```python
from build123d import *

# Parameters (mm, degrees)
SKETCH1_W           = 6.35
SKETCH1_H           = 12.7
BOSS_EXTRUDE1_DEPTH = 2.54
SKETCH2_W           = 6.35
SKETCH2_H           = 0.127
BOSS_EXTRUDE2_DEPTH = 0.254
CUT_EXTRUDE1_DEPTH  = 10.404862359


with BuildPart() as part:
    # Sketch1 → Boss-Extrude1 (new body)
    with BuildSketch(Plane.XY):
        Rectangle(SKETCH1_W, SKETCH1_H)
    extrude(amount=BOSS_EXTRUDE1_DEPTH)

    # Sketch2 → Boss-Extrude2 (add)
    with BuildSketch(Plane.XY.offset(2.54)):
        with Locations((0, -6.2865)):
            Rectangle(SKETCH2_W, SKETCH2_H)
    boss_extrude2 = extrude(amount=BOSS_EXTRUDE2_DEPTH)

    # Mirror1: Boss-Extrude2 across plane
    add(boss_extrude2.mirror(Plane.ZX))

    # Sketch3 → Cut-Extrude1 (cut, through all)
    with BuildSketch(Plane(origin=(3.175, 0, 0), x_dir=(0, 0, -1), z_dir=(1, 0, 0))):
        Polygon((0, -6.35), (-2.286, -6.35), (0, 0), align=None)
    extrude(amount=-CUT_EXTRUDE1_DEPTH, mode=Mode.SUBTRACT)


solid = part.part
```
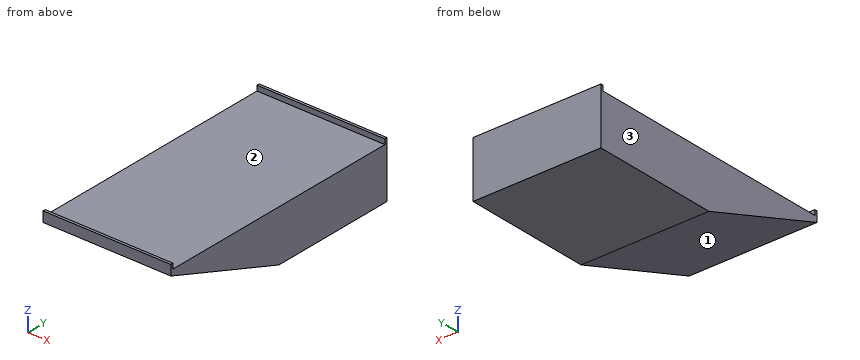
Work out the finished part from the listing and answer in its coordinate system (mm). Face numbers are marked on the shaded views. Round coordinates to 2 decimals unless told otherwise and drop trailing zeros. Loops run counter-clockwise (first coordinate to the right, second up) from the corner with the lowest first, then second, coordinate; pieces in that order, holes last. Notation, with made-up numbers: M 70,-40 L 119,-40 A32 ccw 119,-3 Z; hole C -10.75,0 d2. An arc over 180 degrees is marked long. One line per question, with ' | ' between items.
Q1. Consider line 1 along Z through (x, y) = (1.25, 4.5); line 2 along Z through (x, y) = (2, -4). Determine where each line is inside the solid, lowest interval first. Write a range as from..to.
Conclusion:
line 1: z = 0..2.54 | line 2: z = 1.44..2.54
Q2. Find section C-C, the plane z = 0.45. Give the vertices of the cut face in (x, y) (3 decimals).
Conclusion:
outline: M -3.175,-1.25 L 3.175,-1.25 L 3.175,6.35 L -3.175,6.35 Z
Q3. The mould has two halves that part along Y. Classify the marked faces 1, 2 and 3: +Y half, -Y half, draft (parallel to the pull), parting line (faces both ways), or undercut.
Conclusion:
face 1: -Y half | face 2: undercut | face 3: draft
Q4. Each of these flat-tipped pins is pushed along its axis until it touches: pin 1 Ø1.9 at (x, y) = (-0.5, 1.5) entering from +Z; pin 2 Ø1 at (y, z) = (-4.5, 0.5) entering from +X. Where does it stop, or does it pass through?
Conclusion:
pin 1: stops at z = 2.54 | pin 2: passes through
Q5. Find section A-A, the plane x = 2. Give the vertices of the cut face in (y, z).
Conclusion:
outline: M -6.35,2.29 L 0,0 L 6.35,0 L 6.35,2.79 L 6.22,2.79 L 6.22,2.54 L -6.22,2.54 L -6.22,2.79 L -6.35,2.79 Z
Q6. Find section B-B, the plane y = -1.25. Give the vertices of the cut face in (x, z) (3 decimals).
Conclusion:
outline: M -3.175,0.45 L 3.175,0.45 L 3.175,2.54 L -3.175,2.54 Z
